Here's how the part is built. I have some questions about the finished solid (model axes, mm). A direction names the side the tool comes from. Round coordinates to 2 decimals unless told otherwise and drop trailing zeros. Order: outer loops, then holes, each group sorted by start corner. A loop starts at its lowest first (then second) coordinate and runs counter-clockwise, first axis right, second up. Notation, with made-up numbers: (49, -3.75) -> (73, -3.75) arc R13 ccw to (73, 13.25) -> close; hole circle Ø11 at (-1, -31.5). An arc over 180 degrees is marked (long way). Answer in a Markdown table with one row per item.
```python
from build123d import *

# Parameters (mm, degrees)
F1_W      = 54.708
F1_H      = 77.4
F2_DEPTH  = 11.3
F3_T      = -1.5
F4_W      = 20.1
F4_H      = 17.4
F5_DEPTH  = 6.3
F6_R      = 4.5
F7_DEPTH  = 2.3
F8_R      = 1.5
F9_DEPTH  = 11.301
F10_SIZE  = 1
F11_R     = 1.75
F12_DEPTH = 11.3
F13_R     = 1.5
F14_DEPTH = 2
F15_SIZE  = 1.5
F16_W     = 7.5
F16_H     = 1.5
F17_DEPTH = 6.3


with BuildPart() as f2:
    # F1 (on face) → F2 (new body)
    with BuildSketch(Plane.XY):
        with Locations((25.654, 37)):
            Rectangle(F1_W, F1_H)
    extrude(amount=F2_DEPTH)

    # F3
    f3_openings = [f2.faces().sort_by_distance(p)[0] for p in [
        (25.654, 37, 11.3),
    ]]
    offset(amount=F3_T, openings=f3_openings)

    # F4 (on face) → F5 (cut, through all)
    with BuildSketch(Plane.XY.offset(11.3)):
        with Locations((8.35, 26)):
            Rectangle(F4_W, F4_H)
        with Locations((42.958, 26)):
            Rectangle(F4_W, F4_H)
        with Locations((8.35, 62)):
            Rectangle(F4_W, F4_H)
        with Locations((42.958, 62)):
            Rectangle(F4_W, F4_H)
    extrude(amount=-F5_DEPTH, mode=Mode.SUBTRACT)

    # F6 (on face) → F7 (join, through all)
    with BuildSketch(Plane.XY.offset(1.5)):
        with BuildLine():
            Line((-1.7, 74.8469880528), (-1.7, 69.3930119472))
            ThreePointArc((-1.7, 69.3930119472), (6.3796, 72.12), (-1.7, 74.8469880528))
        make_face()
        with BuildLine():
            Line((53.008, 69.3930119472), (53.008, 74.8469880528))
            ThreePointArc((53.008, 74.8469880528), (44.9284, 72.12), (53.008, 69.3930119472))
        make_face()
        with Locations((11.2141, 3.9243)):
            Circle(F6_R)
        with Locations((32.512, 3.9243)):
            Circle(F6_R)
        with BuildLine():
            Line((53.008, 1.1973119472), (53.008, 6.6512880528))
            ThreePointArc((53.008, 6.6512880528), (44.9284, 3.9243), (53.008, 1.1973119472))
        make_face()
    extrude(amount=F7_DEPTH)

    # F8 (on face) → F9 (cut, through all)
    with BuildSketch(Plane(origin=(0, 0, 0), x_dir=(1, 0, 0), z_dir=(0, 0, -1))):
        with Locations((14.404, -54.75)):
            Circle(F8_R)
        with Locations((14.404, -19.25)):
            Circle(F8_R)
        with Locations((36.904, -19.25)):
            Circle(F8_R)
        with Locations((36.904, -54.75)):
            Circle(F8_R)
    extrude(amount=-F9_DEPTH, mode=Mode.SUBTRACT)

    # F10
    f10_edges = [f2.edges().sort_by_distance(p)[0] for p in [
        (35.404, 54.75, 1.5),
        (12.904, 54.75, 1.5),
        (35.404, 19.25, 1.5),
        (12.904, 19.25, 1.5),
    ]]
    chamfer(f10_edges, length=F10_SIZE)

    # F11 (on face) → F12 (join, through all)
    with BuildSketch(Plane(origin=(0, 0, 0), x_dir=(1, 0, 0), z_dir=(0, 0, -1))):
        with BuildLine():
            Line((-1.7, 1.7), (-6.7, 1.7))
            ThreePointArc((-6.7, 1.7), (-11.7, -3.3), (-6.7, -8.3))
            Line((-6.7, -8.3), (-1.7, -8.3))
            Line((-1.7, -8.3), (-1.7, 1.7))
        make_face()
        with Locations((-6.7, -3.3)):
            Circle(F11_R, mode=Mode.SUBTRACT)
        with BuildLine():
            Line((-1.7, -75.7), (-1.7, -80.7))
            ThreePointArc((-1.7, -80.7), (3.3, -85.7), (8.3, -80.7))
            Line((8.3, -80.7), (8.3, -75.7))
            Line((8.3, -75.7), (-1.7, -75.7))
        make_face()
        with Locations((3.3, -80.7)):
            Circle(F11_R, mode=Mode.SUBTRACT)
        with BuildLine():
            Line((53.008, -8.3), (58.008, -8.3))
            ThreePointArc((58.008, -8.3), (63.008, -3.3), (58.008, 1.7))
            Line((58.008, 1.7), (53.008, 1.7))
            Line((53.008, 1.7), (53.008, -8.3))
        make_face()
        with Locations((58.008, -3.3)):
            Circle(F11_R, mode=Mode.SUBTRACT)
        with BuildLine():
            Line((43.008, -75.7), (43.008, -80.7))
            ThreePointArc((43.008, -80.7), (48.008, -85.7), (53.008, -80.7))
            Line((53.008, -80.7), (53.008, -75.7))
            Line((53.008, -75.7), (43.008, -75.7))
        make_face()
        with Locations((48.008, -80.7)):
            Circle(F11_R, mode=Mode.SUBTRACT)
    extrude(amount=-F12_DEPTH)

    # F13 (on face) → F14 (join)
    with BuildSketch(Plane.XY.offset(3.8)):
        with Locations((49.4284, 3.9243)):
            Circle(F13_R)
        with Locations((32.512, 3.9243)):
            Circle(F13_R)
        with Locations((11.2141, 3.9243)):
            Circle(F13_R)
        with Locations((49.4284, 72.12)):
            Circle(F13_R)
        with Locations((1.8796, 72.12)):
            Circle(F13_R)
    extrude(amount=F14_DEPTH)

    # F15
    f15_edges = [f2.edges().sort_by_distance(p)[0] for p in [
        (47.9284, 3.9243, 5.8),
        (31.012, 3.9243, 5.8),
        (9.7141, 3.9243, 5.8),
        (47.9284, 72.12, 5.8),
        (0.3796, 72.12, 5.8),
    ]]
    chamfer(f15_edges, length=F15_SIZE)

    # F16 (on face) → F17 (cut, through all)
    with BuildSketch(Plane.XY.offset(11.3)):
        with Locations((4.75, -0.95)):
            Rectangle(F16_W, F16_H)
    extrude(amount=-F17_DEPTH, mode=Mode.SUBTRACT)


solid = f2.part
```
1. Suppose I cut it at A-A on y = 19.25. Write out the boundary of the cut face in (x, z), then the cut area to 3 significant figures.
Numbers:
| item | result |
|---|---|
| outline | (-1.7, 0) -> (12.9, 0) -> (12.9, 0.5) -> (11.9, 1.5) -> (-0.2, 1.5) -> (-0.2, 5) -> (-1.7, 5) -> close; (15.9, 0) -> (35.4, 0) -> (35.4, 0.5) -> (34.4, 1.5) -> (16.9, 1.5) -> (15.9, 0.5) -> close; (38.4, 0) -> (53.01, 0) -> (53.01, 5) -> (51.51, 5) -> (51.51, 1.5) -> (39.4, 1.5) -> (38.4, 0.5) -> close |
| area | 81.6 mm2 |
2. For pin 1 Ø3 at (y, z) = (50, 1.5) entering from -X; pin 2 Ø1.2 at (y, z) = (-0.5, 8.5) entering from -X; pin 3 Ø6 at (x, z) = (54.5, 4.5) entering from +Y, each with a flat end and sliding along its axis, tell me the tip position at first contact or that it passes through.
Numbers:
| item | result |
|---|---|
| pin 1 | stops at x = -1.7 |
| pin 2 | stops at x = -10.54 |
| pin 3 | stops at y = 84.28 |
3. Suppose I cut it at D-D on y = 33. Write out the boundary of the cut face in (x, z), then the cut area to 3 significant figures.
Numbers:
| item | result |
|---|---|
| outline | (-1.7, 0) -> (53.01, 0) -> (53.01, 5) -> (51.51, 5) -> (51.51, 1.5) -> (-0.2, 1.5) -> (-0.2, 5) -> (-1.7, 5) -> close |
| area | 92.6 mm2 |
4. Please list where these lines run through material, in increasing order: line 1 along X through (y, z) = (3.3, 8.75); line 2 along Y through (x, z) = (24.5, 10.25); line 3 along Y through (x, z) = (3.3, 6.25).
Numbers:
| item | result |
|---|---|
| line 1 | x = -11.7 to -8.45, -4.95 to -0.2, 51.51 to 56.26, 59.76 to 63.01 |
| line 2 | y = -1.7 to -0.2, 74.2 to 75.7 |
| line 3 | y = 74.2 to 78.95, 82.45 to 85.7 |
5. We'd pull the mould along X, two halves only. Please class faces 1 (the face through (53.008, 44, 4)), 2 (the face through (25, -0.2, 6)), 3 (the face through (55, 8.3, 6)): released by +X, released by -X, zero draft, split by the parting line, or undercut.
Numbers:
| item | result |
|---|---|
| face 1 | released by +X |
| face 2 | undercut |
| face 3 | zero draft |
6. Suppose I cut it at C-C on x = 23. Write out the boundary of the cut face in (y, z).
Numbers:
| item | result |
|---|---|
| outline | (-1.7, 0) -> (75.7, 0) -> (75.7, 11.3) -> (74.2, 11.3) -> (74.2, 1.5) -> (-0.2, 1.5) -> (-0.2, 11.3) -> (-1.7, 11.3) -> close |
7. Suppose I cut it at B-B on z = 7.25. State how many separate pieces and enclosed holes the cut face has, then the cut area to 3 significant figures.
Numbers:
| item | result |
|---|---|
| separate pieces | 5 |
| enclosed holes | 4 |
| area | 590 mm2 |
8. For faces 4 (the face through (47.9, 85.7, 5.6)), 5 (the face through (33.898, 3.35, 4.046)), which set-ups out of +Z, -Z, +X, -X, +Y, -Y let a thin tool reach every point of the face, with its end or its side?
Numbers:
| item | result |
|---|---|
| face 4 | +Z, -Z, +Y |
| face 5 | +Z |
